Build history of the part. All positions in model axes, mm. A direction names the side the tool comes from. Give positions to 0.01 mm unless a question says otherwise; leave off trailing zeros. Loops run counter-clockwise (first coordinate to the right, second up) from the corner with the lowest first, then second, coordinate; pieces in that order, holes last. Notation, with made-up numbers: M -38.75,5 L 3.25,5 A25 cw 3.25,20 Z; hole C 1.25,-21 d2. An arc over 180 degrees is marked long. Put each result on its own line as item: value.
```python
from build123d import *

# Parameters (mm, degrees)
F1_DEPTH = 4.5
F2_R     = 1
F4_DEPTH = 4
F5_W     = 12.5
F5_H     = 2.9783394848
F6_DEPTH = 3.1


with BuildPart() as f1:
    # F0 (on Top) → F1 (new body)
    with BuildSketch(Plane.XY):
        with BuildLine():
            ThreePointArc((0, 3.8761399509), (0.2928932188, 3.1690331698), (1, 2.8761399509))
            Line((1, 2.8761399509), (29, 2.8761399509))
            ThreePointArc((29, 2.8761399509), (29.7071067812, 3.1690331698), (30, 3.8761399509))
            Line((30, 3.8761399509), (30, 13.8761399509))
            ThreePointArc((30, 13.8761399509), (29.7071067812, 14.5832467321), (29, 14.8761399509))
            Line((29, 14.8761399509), (1, 14.8761399509))
            ThreePointArc((1, 14.8761399509), (0.2928932188, 14.5832467321), (0, 13.8761399509))
            Line((0, 13.8761399509), (0, 3.8761399509))
        make_face()
        with BuildLine():
            ThreePointArc((5, 8.6761399509), (5.2928932188, 9.3832467321), (6, 9.6761399509))
            Line((6, 9.6761399509), (12.5, 9.6761399509))
            ThreePointArc((12.5, 9.6761399509), (13.2071067812, 9.3832467321), (13.5, 8.6761399509))
            Line((13.5, 8.6761399509), (13.5, 7.8761399509))
            ThreePointArc((13.5, 7.8761399509), (13.2071067812, 7.1690331698), (12.5, 6.8761399509))
            Line((12.5, 6.8761399509), (6, 6.8761399509))
            ThreePointArc((6, 6.8761399509), (5.2928932188, 7.1690331698), (5, 7.8761399509))
            Line((5, 7.8761399509), (5, 8.6761399509))
        make_face(mode=Mode.SUBTRACT)
    extrude(amount=F1_DEPTH)

    # F2
    f2_edges = [f1.edges().sort_by_distance(p)[0] for p in [
        (0.292893, 3.169033, 4.5),
        (15, 2.87614, 4.5),
        (29.707107, 3.169033, 4.5),
        (30, 8.87614, 4.5),
        (29.707107, 14.583247, 4.5),
        (15, 14.87614, 4.5),
        (0.292893, 14.583247, 4.5),
        (0, 8.87614, 4.5),
        (5.292893, 9.383247, 4.5),
        (9.25, 9.67614, 4.5),
        (13.207107, 9.383247, 4.5),
        (13.5, 8.27614, 4.5),
        (13.207107, 7.169033, 4.5),
        (9.25, 6.87614, 4.5),
        (5.292893, 7.169033, 4.5),
        (5, 8.27614, 4.5),
    ]]
    fillet(f2_edges, radius=F2_R)

    # F3 (on Top) → F4 (cut)
    with BuildSketch(Plane.XY):
        Polygon((28, 3.3761399509), (28, 14.3761399509), (2, 14.3761399509), (2, 3.3761399509), (14.5, 3.3761399509), (27, 3.3761399509), align=None)
    extrude(amount=F4_DEPTH, mode=Mode.SUBTRACT)

    # F5 (on Top) → F6 (cut)
    with BuildSketch(Plane.XY):
        with Locations((21.25, 14.7778680548)):
            Rectangle(F5_W, F5_H)
    extrude(amount=F6_DEPTH, mode=Mode.SUBTRACT)


solid = f1.part
```
Q1. Tool access for faces 4 (the flat face through (9, 14.376, 2)), 5 (the flat face through (12, 14.876, 2)), 6 (the cylindrical face through (9.296, 10.17, 4.362)): list every direction of +Z, -Z, +X, -X, +Y, -Y with a clear straight run to the whole face (end or side of a thin tool).
Here are the results:
face 4: -Z
face 5: +Z, -Z, +X, -X, +Y
face 6: +Z
Q2. Probe line 1 (X direction, y = 9.25, z = 2.45); line 2 (Y direction, x = 14.5, z = 3.2); line 3 (Y direction, x = 21, z = 2.05). List the from-to ranges inside material, lowest first. Write a range as from..to.
Here are the results:
line 1: 0..2, 28..30
line 2: 2.88..3.38, 14.38..14.88
line 3: 2.88..3.38
Q3. Drop flat-ended pins along their axis: pin 1 Ø5.5 at (x, y) = (9, 11) entering from -Z; pin 2 Ø0.6 at (x, y) = (21, 14.5) entering from -Z. Give the stop position or say it passes through.
Here are the results:
pin 1: z = 4
pin 2: z = 3.1
Q4. Mould opens along X. For faces 1 (the flat face through (0, 9, 2)), 2 (the cylindrical face through (29.71, 14.58, 1.73)), 3 (the cylindrical face through (9.205, 6.382, 4.362)) say: pulls with the +X half, pulls with the -X half, needs draft (parallel to the pull), parting line crosses it, or undercut.
Here are the results:
face 1: pulls with the -X half
face 2: pulls with the +X half
face 3: undercut
Q5. Slice it at A-A (z = 2.2). List the corners of the cut face in (x, y), and give its area (3 significant figures).
Here are the results:
outline: M 0,3.88 A1 ccw 1,2.88 L 29,2.88 A1 ccw 30,3.88 L 30,13.88 A1 ccw 29,14.88 L 27.5,14.88 L 27.5,14.38 L 28,14.38 L 28,3.38 L 2,3.38 L 2,14.38 L 15,14.38 L 15,14.88 L 1,14.88 A1 ccw 0,13.88 Z
area: 66.9 mm²
Q6. Slice it at B-B (y = 13.5). List the corners of the cut face in (x, z), and give its area (3 significant figures).
Here are the results:
outline: M 0,0 L 2,0 L 2,4 L 28,4 L 28,0 L 30,0 L 30,3.5 A1 ccw 29,4.5 L 1,4.5 A1 ccw 0,3.5 Z
area: 30.6 mm²
Q7. Slice it at C-C (x = 2.5). List the corners of the cut face in (y, z), and give its area (3 significant figures).
Here are the results:
outline: M 2.88,0 L 3.38,0 L 3.38,4 L 14.38,4 L 14.38,0 L 14.88,0 L 14.88,3.5 A1 ccw 13.88,4.5 L 3.88,4.5 A1 ccw 2.88,3.5 Z
area: 9.57 mm²
